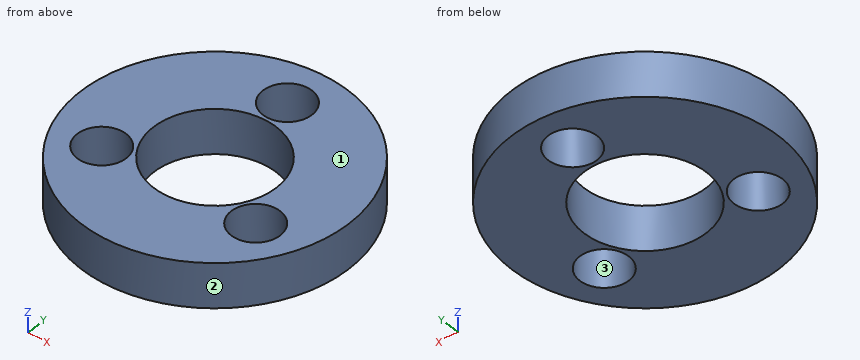
from build123d import *

# Parameters (mm, degrees)
SKETCH1_R            = 6
SKETCH1_R_2          = 2.75
BOSS_EXTRUDE1_DEPTH  = 2
M2_CLEARANCE_HOLE1_D = 2.2


with BuildPart() as part:
    # Sketch1 → Boss-Extrude1 (new body)
    with BuildSketch(Plane.XY):
        with Locations((-27.5, 59.99791663)):
            Circle(SKETCH1_R)
        with Locations((-27.5, 59.99791663)):
            Circle(SKETCH1_R_2, mode=Mode.SUBTRACT)
    extrude(amount=-BOSS_EXTRUDE1_DEPTH)

    # M2 Clearance Hole1 (through all)
    with Locations(Plane.XY):
        with Locations((-27.5, 63.99791663), (-24.035898385, 57.99791663), (-30.964101615, 57.99791663)):
            Hole(M2_CLEARANCE_HOLE1_D / 2)


solid = part.part
The listing builds one solid part. Answer for the finished solid, in the listing's coordinates (mm). Face numbers are marked on the shaded views. Give positions to 0.01 mm unless a question says otherwise; leave off trailing zeros. Order: outer loops, then holes, each group sorted by start corner. A loop starts at its lowest first (then second) coordinate and runs counter-clockwise, first axis right, second up. Notation, with made-up numbers: (72, 10) - (93, 10) arc R17 ccw to (93, 20) - close; hole circle Ø5 at (0, 85.25). An arc over 180 degrees is marked (long way). One line per item, written item: value. Start each with the question number.
1) A cutting plane is placed at A-A on x = -27.5. Give the vertices of the cut face in (y, z), then the cut area to 3 significant figures.
2) Find the intervals of material crossed by L1, parallel to Y at x = -27.5, z = -1.25; L2, parallel to X at y = 60, z = -1.2; L3, parallel to X at y = 57, z = -1.6, in increasing order.
3) Given pin 1 Ø2 at (x, y) = (-24.04, 58) entering from -Z, flat-ended and moving along its own axis, determine where the tip first touches the part or whether it passes through.
4) A cutting plane is placed at D-D on z = -0.25. Give the vertices of the cut face in (x, y).
5) The mould has two halves that part along X. Classify the marked faces 1, 2 and 3: released by +X, released by -X, zero draft, split by the parting line, or undercut.
6) A cutting plane is placed at B-B on y = 63.75. Give the vertices of the cut face in (x, z), then the cut area to 3 significant figures.
7) A cutting plane is placed at C-C on x = -25.75. Give the vertices of the cut face in (y, z).
Answer sheet:
1. outline: (54, -2) - (57.25, -2) - (57.25, 0) - (54, 0) - close; (62.75, -2) - (62.9, -2) - (62.9, 0) - (62.75, 0) - close; (65.1, -2) - (66, -2) - (66, 0) - (65.1, 0) - close
1. area: 8.60 mm2
2. L1: y = 54 to 57.25, 62.75 to 62.9, 65.1 to 66
2. L2: x = -33.5 to -30.25, -24.75 to -21.5
2. L3: x = -32.7 to -31.43, -30.5 to -24.5, -23.57 to -22.3
3. pin 1: passes through
4. outline: circle Ø12 at (-27.5, 60); hole circle Ø2.2 at (-30.96, 58); hole circle Ø5.5 at (-27.5, 60); hole circle Ø2.2 at (-27.5, 64); hole circle Ø2.2 at (-24.04, 58)
5. face 1: zero draft
5. face 2: split by the parting line
5. face 3: undercut
6. outline: (-32.18, -2) - (-28.57, -2) - (-28.57, 0) - (-32.18, 0) - close; (-26.43, -2) - (-22.82, -2) - (-22.82, 0) - (-26.43, 0) - close
6. area: 14.4 mm2
7. outline: (54.26, -2) - (57.88, -2) - (57.88, 0) - (54.26, 0) - close; (62.12, -2) - (65.74, -2) - (65.74, 0) - (62.12, 0) - close
